Here's the drawing with two shaded views (mm, measured from the low corner). I have some questions. Round coordinates to 2 decimals unless told otherwise and drop trailing zeros. Order: outer loops, then holes, each group sorted by start corner. A loop starts at its lowest first (then second) coordinate and runs counter-clockwise, first axis right, second up. Notation, with made-up numbers: M 6,51 L 43,51 A19 cw 43,68 Z; hole C 46,-20 d8. An arc over 180 degrees is marked long. One line per question, with ' | ' between items.
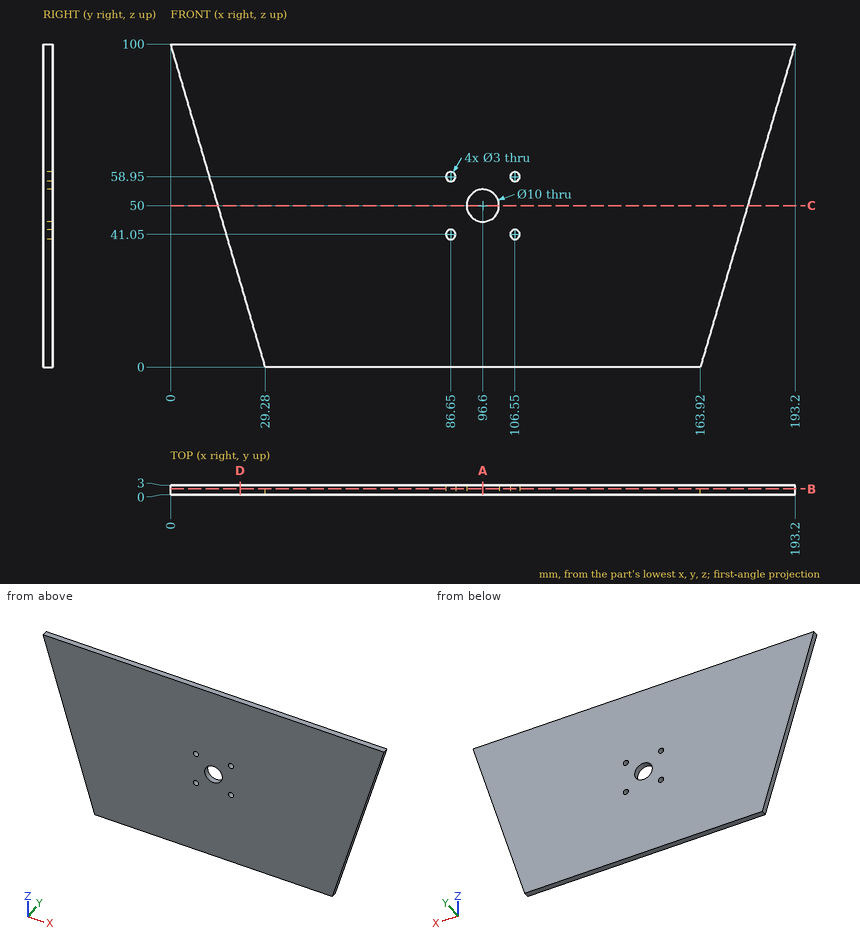
(1) Please list where these lines run through material, in increasing order: probe 1 along Z at (x, y) = (106.55, 1.7); probe 2 along X at (y, z) = (1.2, 40.5); probe 3 along Z at (x, y) = (96.6, 0.95). Write a range as [from, to].
Final values:
probe 1: [0, 39.55], [42.55, 57.45], [60.45, 100] | probe 2: [17.42, 85.25], [88.05, 105.15], [107.95, 175.78] | probe 3: [0, 45], [55, 100]
(2) If we section it at B-B on y = 1.85: Please give me the cut outline in (x, z), plus the area to 3 significant figures.
Final values:
outline: M 0,100 L 29.28,0 L 163.92,0 L 193.2,100 Z; hole C 86.65,41.05 d3; hole C 86.65,58.95 d3; hole C 96.6,50 d10; hole C 106.55,41.05 d3; hole C 106.55,58.95 d3 | area: 16,300 mm^2
(3) If we section it at C-C on z = 50: Please give me the cut outline in (x, y).
Final values:
outline: M 14.64,0 L 91.6,0 L 91.6,3 L 14.64,3 Z; M 101.6,0 L 178.56,0 L 178.56,3 L 101.6,3 Z
(4) If we section it at A-A on x = 96.6: Please give me the cut outline in (y, z).
Final values:
outline: M 0,0 L 3,0 L 3,45 L 0,45 Z; M 0,55 L 3,55 L 3,100 L 0,100 Z
(5) If we section it at D-D on x = 21.5: Please give me the cut outline in (y, z).
Final values:
outline: M 0,26.57 L 3,26.57 L 3,100 L 0,100 Z
(6) Will these pins go through, and if not, where does the flat tip stop? pin 1 Ø8 at (x, z) = (96.6, 50) entering from +Y; pin 2 Ø1.5 at (x, z) = (119.5, 32) entering from -Y.
Final values:
pin 1: through | pin 2: y = 0
